Can you work these out from the model? Positions are in its coordinate system, mm. Face numbers are marked on the shaded views. A direction names the side the tool comes from. Give positions to 0.01 mm unless a question says otherwise; leave off trailing zeros. Loops run counter-clockwise (first coordinate to the right, second up) from the corner with the lowest first, then second, coordinate; pieces in that order, holes last. Notation, with made-up numbers: (61.25, 40) -> (116.25, 40) arc R24 ccw to (116.25, 78) -> close; hole circle Ø10 at (-15.5, 57). An arc over 180 degrees is marked (long way). Use CSV: the item, a comma, the result in double quotes.
from build123d import *

# Parameters (mm, degrees)
SKETCH4_W           = 106
SKETCH4_H           = 170
BOSS_EXTRUDE4_DEPTH = 10
SKETCH5_W           = 106
SKETCH5_H           = 20
BOSS_EXTRUDE5_DEPTH = 60
SKETCH6_W           = 106
SKETCH6_H           = 1.75
CUT_EXTRUDE2_DEPTH  = 40
SKETCH7_R           = 4.15
CUT_EXTRUDE3_DEPTH  = 40
SKETCH8_W           = 106
SKETCH8_H           = 60
CUT_EXTRUDE4_DEPTH  = 40


with BuildPart() as part:
    # Sketch4 → Boss-Extrude4 (new body)
    with BuildSketch(Plane(origin=(0, 0, 0), x_dir=(1, 0, 0), z_dir=(0, 1, 0))):
        Rectangle(SKETCH4_W, SKETCH4_H)
    extrude(amount=BOSS_EXTRUDE4_DEPTH)

    # Sketch5 → Boss-Extrude5 (add)
    with BuildSketch(Plane(origin=(0, 10, 0), x_dir=(1, 0, 0), z_dir=(0, 1, 0))):
        with Locations((0, 75)):
            Rectangle(SKETCH5_W, SKETCH5_H)
        with Locations((0, -75)):
            Rectangle(SKETCH5_W, SKETCH5_H)
    extrude(amount=BOSS_EXTRUDE5_DEPTH)

    # Sketch6 → Cut-Extrude2 (cut)
    with BuildSketch(Plane.XY.offset(85)):
        with Locations((0, 5)):
            Rectangle(SKETCH6_W, SKETCH6_H)
    extrude(amount=-CUT_EXTRUDE2_DEPTH, mode=Mode.SUBTRACT)

    # Sketch7 → Cut-Extrude3 (cut)
    with BuildSketch(Plane(origin=(0, 10, 0), x_dir=(1, 0, 0), z_dir=(0, 1, 0))):
        with Locations(Location((0, -55, 0), (0, 0, 90))):
            Circle(SKETCH7_R)
        with Locations(Location((30, -55, 0), (0, 0, 90))):
            Circle(SKETCH7_R)
        with Locations(Location((-30, -55, 0), (0, 0, 90))):
            Circle(SKETCH7_R)
    extrude(amount=-CUT_EXTRUDE3_DEPTH, mode=Mode.SUBTRACT)

    # Sketch8 → Cut-Extrude4 (cut)
    with BuildSketch(Plane(origin=(0, 0, 65), x_dir=(-1, 0, 0), z_dir=(0, 0, -1))):
        with Locations((0, 40)):
            Rectangle(SKETCH8_W, SKETCH8_H)
    extrude(amount=-CUT_EXTRUDE4_DEPTH, mode=Mode.SUBTRACT)


solid = part.part
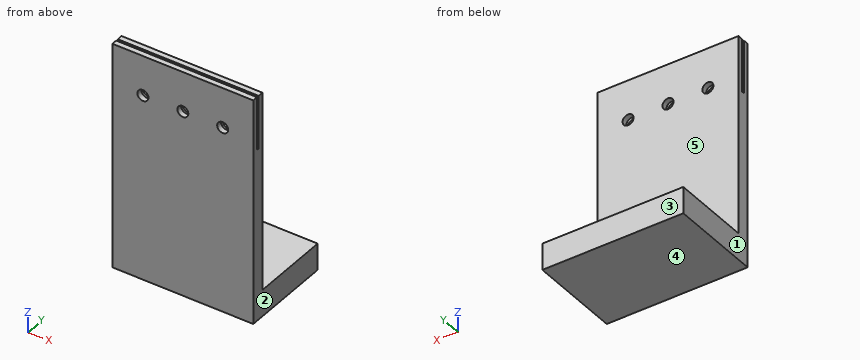
(1) If we section it at B-B, the plane z = 55: Give the number of separate pieces and of enclosed holes in the cut face, then the cut area to 3 significant figures.
Answer sheet:
separate pieces,"8"
enclosed holes,"0"
area,"669 mm2"
(2) Which directions (+Z, -Z, +X, -X, +Y, -Y) give clear straight access to the entire face, cutting with the end or side of a thin tool? Please do the marked faces 4 and 5.
Answer sheet:
face 4,"-Z, +X, -X, +Y, -Y"
face 5,"+Z, +X, -X, +Y"
(3) Will these pins go through, and if not, where does the flat tip stop? pin 1 Ø10 at (x, z) = (-25.5, -24.5) entering from -Y; pin 2 Ø1 at (x, y) = (30, 16.5) entering from +Z; pin 3 Ø9.5 at (x, z) = (-30, 55) entering from +Y.
Answer sheet:
pin 1,"stops at y = 0"
pin 2,"stops at z = -65"
pin 3,"stops at y = 10"
(4) We'd pull the mould along X, two halves only. Please class the marked faces 1, 2 and 3: released by +X, released by -X, zero draft, split by the parting line, or undercut.
Answer sheet:
face 1,"released by -X"
face 2,"released by +X"
face 3,"zero draft"
(5) If we section it at C-C, the plane x = -37.5: Write out the boundary of the cut face in (y, z) (3 decimals), then the cut area to 3 significant figures.
Answer sheet:
outline,"(0, -85) -> (70, -85) -> (70, -65) -> (10, -65) -> (10, 85) -> (5.875, 85) -> (5.875, 45) -> (4.125, 45) -> (4.125, 85) -> (0, 85) -> close"
area,"2,830 mm2"
(6) If we section it at D-D, the plane y = 60: Write out the boundary of the cut face in (x, z).
Answer sheet:
outline,"(-53, -85) -> (53, -85) -> (53, -65) -> (-53, -65) -> close"
(7) If we section it at A-A, the plane x = 30: Write out the boundary of the cut face in (y, z) (3 decimals).
Answer sheet:
outline,"(0, -85) -> (70, -85) -> (70, -65) -> (10, -65) -> (10, 50.85) -> (5.875, 50.85) -> (5.875, 45) -> (4.125, 45) -> (4.125, 50.85) -> (0, 50.85) -> close; (0, 59.15) -> (4.125, 59.15) -> (4.125, 85) -> (0, 85) -> close; (5.875, 59.15) -> (10, 59.15) -> (10, 85) -> (5.875, 85) -> close"
(8) If I drill on L1, parallel to X at y = 2.15, z = 55; L2, parallel to Y at x = 7, z = 60.5 (3 decimals); L3, parallel to Z at x = 30.5, y = 9, over which ranges is the centre line in solid material (lowest first)? Write a range as from..to.
Answer sheet:
L1,"x = -53..-34.15, -25.85..-4.15, 4.15..25.85, 34.15..53"
L2,"y = 0..4.125, 5.875..10"
L3,"z = -85..50.88, 59.12..85"
